The model under review builds one solid part; all positions refer to its coordinate system, in mm. A direction names the side the tool comes from. Give positions to 0.01 mm unless a question says otherwise; leave off trailing zeros. Order: outer loops, then holes, each group sorted by start corner. A loop starts at its lowest first (then second) coordinate and runs counter-clockwise, first axis right, second up. Notation, with made-up numbers: (88.25, 61.25) - (97.25, 61.25) arc R20 cw to (97.25, 82.25) - close; hole circle Ø7 at (43.25, 0). An arc over 180 degrees is marked (long way). Use a Markdown table: item, result. Add a question column.
```python
from build123d import *

# Parameters (mm, degrees)
F0_R     = 26
F0_R_2   = 8.875
F0_R_3   = 4.25
F1_DEPTH = 5


with BuildPart() as f1:
    # F0 (on Top) → F1 (new body)
    with BuildSketch(Plane.XY):
        Circle(F0_R)
        with BuildLine():
            ThreePointArc((-11.074626, -15.663465), (-16.970563, -16.970563), (-15.663465, -11.074626))
            Line((-15.663465, -11.074626), (-8.448647, -8.448647))
            Line((-8.448647, -8.448647), (-11.074626, -15.663465))
        make_face(mode=Mode.SUBTRACT)
        with Locations((0, -15.125)):
            Circle(F0_R_2, mode=Mode.SUBTRACT)
        with BuildLine():
            Line((11.074626, -15.663465), (8.448647, -8.448647))
            Line((8.448647, -8.448647), (15.663465, -11.074626))
            ThreePointArc((15.663465, -11.074626), (17.371712, -12.385409), (18.019191, -14.438951))
            ThreePointArc((18.019191, -14.438951), (15.060653, -17.964799), (11.074626, -15.663465))
        make_face(mode=Mode.SUBTRACT)
        with Locations((-15.125, 0)):
            Circle(F0_R_2, mode=Mode.SUBTRACT)
        with BuildLine():
            ThreePointArc((-15.663465, 11.074626), (-16.970563, 16.970563), (-11.074626, 15.663465))
            Line((-11.074626, 15.663465), (-8.448647, 8.448647))
            Line((-8.448647, 8.448647), (-15.663465, 11.074626))
        make_face(mode=Mode.SUBTRACT)
        Circle(F0_R_3, mode=Mode.SUBTRACT)
        with Locations((15.125, 0)):
            Circle(F0_R_2, mode=Mode.SUBTRACT)
        with Locations((0, 15.125)):
            Circle(F0_R_2, mode=Mode.SUBTRACT)
        with BuildLine():
            Line((15.663465, 11.074626), (8.448647, 8.448647))
            Line((8.448647, 8.448647), (11.074626, 15.663465))
            ThreePointArc((11.074626, 15.663465), (15.060653, 17.964799), (18.019191, 14.438951))
            ThreePointArc((18.019191, 14.438951), (17.371712, 12.385409), (15.663465, 11.074626))
        make_face(mode=Mode.SUBTRACT)
    extrude(amount=F1_DEPTH)


solid = f1.part
```
Q1. Machinability: for faces 1 (the flat face through (9.78, -12.11, 2.46)), 2 (the flat face through (-2, 4, 0)), which of the approach directions +Z, -Z, +X, -X, +Y, -Y give a long, thin tool a straight path to every point of the face, cutting with its end or side? Answer none if there is none.
Q2. Draft analysis for pull direction Y (two halves, no side actions). For faces 3 (the cylindrical face through (2.285, 3.584, 2.465)), 4 (the cylindrical face through (-20.633, -15.821, 2.465)), 5 (the flat face through (-12.11, -9.78, 2.46)), 6 (the flat face through (-2, 4, 5)), state which applies: pulls with the +Y half, pulls with the -Y half, needs draft (parallel to the pull), parting line crosses it, or undercut.
Q3. We need section B-B (y = 7.5). Write out the cut boundary in (x, z), plus the area to 3 significant figures.
Q4. Clearance check with flat-ended pins moving along their axes: P1, Ø1.5, axis at y = 19, z = 3, coming from the -X side; P2, Ø1.5, axis at y = 2.5, z = 1, coming from the -X side. State where each tip first meets the part, or that it passes through.
Q5. Wall thickness on probe 1 along Y at (x, z) = (0, 3.95); probe 2 along Y at (x, z) = (-5, 2.7); probe 3 along X at (y, z) = (16, 1.55): over which ranges is each line inside the solid? List them lowest first.
Q6. We need section C-C (y = -5). Write out the cut boundary in (x, z).
Q7. We need section A-A (x = 0). Write out the cut boundary in (y, z).
Here are the results:
| question | item | result |
|---|---|---|
| 1 | face 1 | +Z, -Z |
| 1 | face 2 | -Z, +X, -X, +Y, -Y |
| 2 | face 3 | undercut |
| 2 | face 4 | parting line crosses it |
| 2 | face 5 | undercut |
| 2 | face 6 | needs draft |
| 3 | outline | (-24.89, 0) - (-19.87, 0) - (-19.87, 5) - (-24.89, 5) - close; (-10.38, 0) - (-4.54, 0) - (-4.54, 5) - (-10.38, 5) - close; (4.54, 0) - (10.38, 0) - (10.38, 5) - (4.54, 5) - close; (19.87, 0) - (24.89, 0) - (24.89, 5) - (19.87, 5) - close |
| 3 | area | 109 mm2 |
| 4 | P1 | x = -18.52 |
| 4 | P2 | x = -25.94 |
| 5 | probe 1 | -26 to -24, -6.25 to -4.25, 4.25 to 6.25, 24 to 26 |
| 5 | probe 2 | -25.51 to -22.46, -7.79 to 7.79, 22.46 to 25.51 |
| 5 | probe 3 | -20.49 to -17.66, -11.22 to -8.83, 8.83 to 11.22, 17.66 to 20.49 |
| 6 | outline | (-25.51, 0) - (-22.46, 0) - (-22.46, 5) - (-25.51, 5) - close; (-7.79, 0) - (7.79, 0) - (7.79, 5) - (-7.79, 5) - close; (22.46, 0) - (25.51, 0) - (25.51, 5) - (22.46, 5) - close |
| 7 | outline | (-26, 0) - (-24, 0) - (-24, 5) - (-26, 5) - close; (-6.25, 0) - (-4.25, 0) - (-4.25, 5) - (-6.25, 5) - close; (4.25, 0) - (6.25, 0) - (6.25, 5) - (4.25, 5) - close; (24, 0) - (26, 0) - (26, 5) - (24, 5) - close |
